Part model, mm, in its own coordinate system. A direction names the side the tool comes from. Round coordinates to 2 decimals unless told otherwise and drop trailing zeros. Write each loop counter-clockwise with the first axis right and the second up, starting at its lowest first coordinate (ties: lowest second). Pieces come first, ordered by that corner, then holes. Notation, with made-up numbers: M 25.5,24.5 L 60.5,24.5 A11 cw 60.5,42.5 Z; hole C 24,-20 d1. An arc over 180 degrees is marked long. One line per question, with ' | ' between items. Start each with the question number.
1) Wall check: probe 1 along Y at (x, z) = (0, 0.85); probe 2 along Z at (x, y) = (-2, -10); probe 3 along Y at (x, z) = (0, -7). Give the ranges that are in metal, low to high. Write a range as [from, to].
2) Saw through at C-C (z = -3.5). List the corners of the cut face in (x, y), plus the area to 3 significant figures.
3) Saw through at A-A (y = 0). Give the number of separate pieces and of enclosed holes in the cut face, plus the area to 4 significant figures.
4) Mould opens along X. For faces 1 (the face through (0, -5, 5)), 2 (the face through (-14.6, 13.3, 1)), 3 (the face through (0.867, -3.905, -5.133)), 4 (the face through (-11.253, 0.121, 0.986)) say: pulls with the +X half, pulls with the -X half, needs draft (parallel to the pull), parting line crosses it, or undercut.
5) Drop flat-ended pins along their axis: pin 1 Ø1.5 at (x, z) = (-4, -4.5) entering from -Y; pin 2 Ø6 at (x, z) = (-4.5, -5.5) entering from +Y; pin 3 Ø1 at (x, z) = (-2.5, -7.5) entering from +Y; pin 4 Ø19 at (x, y) = (0.5, -4) entering from -Z. Give the stop position or say it passes through.
6) Tool access for faces 5 (the face through (5, 0, -15)), 6 (the face through (-1.73, 7.81, -7.35)), 7 (the face through (-1.73, -7.81, 3.23)): list every direction of +Z, -Z, +X, -X, +Y, -Y with a clear straight run to the whole face (end or side of a thin tool).
```python
from build123d import *

# Parameters (mm, degrees)
SKETCH_1_R              = 19.75
EXTRUDE_1_DEPTH         = 2
SKETCH_2_R              = 8
EXTRUDE_2_DEPTH         = 3
EXTRUDE_START           = 15
SKETCH_3_R              = 8
EXTRUDE_3_DEPTH         = 15
HOLE_WIZARD_M8_1_D      = 8
HOLE_WIZARD_5_5_5_5_1_D = 5.5
CHAMFER_1_SIZE          = 0.5


with BuildPart() as part:
    # 草图1 → 凸台-拉伸1 (new body)
    with BuildSketch(Plane.XY):
        Circle(SKETCH_1_R)
    extrude(amount=EXTRUDE_1_DEPTH)

    # 草图2 → 凸台-拉伸2 (add)
    with BuildSketch(Plane.XY.offset(2)):
        Circle(SKETCH_2_R)
    extrude(amount=EXTRUDE_2_DEPTH)

    # 草图3 → 凸台-拉伸3 (add)
    with BuildSketch(Plane(origin=(0, 0, 0), x_dir=(-1, 0, 0), z_dir=(0, 0, -1)).offset(EXTRUDE_START)):
        with Locations(Location((0, 0, 0), (0, 0, 180))):
            Circle(SKETCH_3_R)
    extrude(amount=-EXTRUDE_3_DEPTH)

    # M8 螺纹孔1 (through all)
    with Locations(Plane.XY.offset(5)):
        with Locations((0, 0)):
            Hole(HOLE_WIZARD_M8_1_D / 2)

    # Ø5.5 (5.5) 直径孔1 (through all)
    with Locations(Plane.XY.offset(2)):
        with Locations((0, 14), (0, -14), (-14, 0), (14, 0)):
            Hole(HOLE_WIZARD_5_5_5_5_1_D / 2)

    # 倒角1
    chamfer_1_edges = [part.edges().sort_by_distance(p)[0] for p in [
        (-8, 0, -15),
        (4, 0, 5),
        (4, 0, -15),
        (-19.75, 0, 0),
        (-19.75, 0, 2),
        (-8, 0, 5),
    ]]
    chamfer(chamfer_1_edges, length=CHAMFER_1_SIZE)


solid = part.part
```
Answer key:
1) probe 1: y = [-19.75, -16.75], [-11.25, -4], [4, 11.25], [16.75, 19.75] | probe 2: z = [0, 2] | probe 3: y = [-8, -4], [4, 8]
2) outline: C 0,0 d16; hole C 0,0 d8 | area: 151 mm2
3) separate pieces: 4 | enclosed holes: 0 | area: 183.5 mm2
4) face 1: needs draft | face 2: parting line crosses it | face 3: undercut | face 4: undercut
5) pin 1: stops at y = -7.31 | pin 2: stops at y = 7.86 | pin 3: stops at y = 7.75 | pin 4: stops at z = -15
6) face 5: -Z, +X, -X, +Y, -Y | face 6: -Z | face 7: +Z
